from build123d import *

# Parameters (mm, degrees)
BOSS_EXTRU_1_DEPTH = 5
ESQUISSE2_R        = 5
BOSS_EXTRU_2_DEPTH = 15


with BuildPart() as part:
    # Esquisse1 → Boss.-Extru.1 (new body)
    with BuildSketch(Plane(origin=(0, 0, 0), x_dir=(1, 0, 0), z_dir=(0, 1, 0))):
        with BuildLine():
            Line((-4, 0), (-166, 0))
            ThreePointArc((-166, 0), (-168.828427125, 1.171572875), (-170, 4))
            Line((-170, 4), (-170, 6))
            ThreePointArc((-170, 6), (-168.828427125, 8.828427125), (-166, 10))
            Line((-166, 10), (-4, 10))
            ThreePointArc((-4, 10), (-1.171572875, 8.828427125), (0, 6))
            Line((0, 6), (0, 4))
            ThreePointArc((0, 4), (-1.171572875, 1.171572875), (-4, 0))
        make_face()
    extrude(amount=BOSS_EXTRU_1_DEPTH)

    # Esquisse2 → Boss.-Extru.2 (add)
    with BuildSketch(Plane(origin=(0, 5, 0), x_dir=(1, 0, 0), z_dir=(0, 1, 0))):
        with Locations((-160, 5)):
            Circle(ESQUISSE2_R)
        with Locations((-85, 5)):
            Circle(ESQUISSE2_R)
        with Locations((-10, 5)):
            Circle(ESQUISSE2_R)
    extrude(amount=BOSS_EXTRU_2_DEPTH)


solid = part.part
Can you work these out from the model? Positions are in its coordinate system, mm. A direction names the side the tool comes from. Give positions to 0.01 mm unless a question says otherwise; leave off trailing zeros. Order: outer loops, then holes, each group sorted by start corner. A loop starts at its lowest first (then second) coordinate and runs counter-clockwise, first axis right, second up. Notation, with made-up numbers: M -29.5,84.25 L -4.5,84.25 A11 ccw -4.5,95.25 Z; hole C 1.5,78.5 d2. An arc over 180 degrees is marked long. One line per item, written item: value.
Item 1: For faces 4 (the face through (-166, 5, -5)), 5 (the face through (-1.141, 2.465, -1.203)), 6 (the face through (-164, 12, -2)), which set-ups out of +Z, -Z, +X, -X, +Y, -Y let a thin tool reach every point of the face, with its end or its side?
Verdict:
face 4: -X, +Y
face 5: +Z, +X, +Y, -Y
face 6: +Y
Item 2: If we mould it in two halves opening along X, with no side actions, what happens to faces 1 (the face through (-122, 5, -5)), 2 (the face through (-86, 2, -10)), 3 (the face through (-168.797, 2.465, -1.141))? For each: pulls with the +X half, pulls with the -X half, needs draft (parallel to the pull), parting line crosses it, or undercut.
Verdict:
face 1: undercut
face 2: needs draft
face 3: pulls with the -X half
Item 3: If we section it at A-A on y = 15.5: Write out the boundary of the cut face in (x, z).
Verdict:
outline: C -160,-5 d10; C -85,-5 d10; C -10,-5 d10
Item 4: If we section it at B-B on x = -121.5: Write out the boundary of the cut face in (y, z).
Verdict:
outline: M 0,-10 L 5,-10 L 5,0 L 0,0 Z
Item 5: Please list where these lines run through material, in increasing order: line 1 (X direction, y = 17.75, z = -5.25); line 2 (X direction, y = 12.25, z = -1.25); line 3 (Y direction, x = -25.5, z = -4).
Verdict:
line 1: -164.99 to -155.01, -89.99 to -80.01, -14.99 to -5.01
line 2: -163.31 to -156.69, -88.31 to -81.69, -13.31 to -6.69
line 3: 0 to 5
Item 6: For pin 1 (5 mm diameter, centred on x = -42.5, z = -5, fed in from +Y); pin 2 (5 mm diameter, centred on x = -166.5, z = -7, fed in from +Y); pin 3 (1.5 mm diameter, centred on y = 10, z = -7.5, fed in from -X); pin 4 (1 mm diameter, centred on y = 6.5, z = -7, fed in from +X), each with a flat end and sliding along its axis, tell me the tip position at first contact or that it passes through.
Verdict:
pin 1: y = 5
pin 2: y = 20
pin 3: x = -164.68
pin 4: x = -5.23
